Study the drawing (mm; zero at the part's minimum x, y, z) and answer. Round coordinates to 2 decimals unless told otherwise and drop trailing zeros. Write each loop counter-clockwise with the first axis right and the second up, starting at its lowest first coordinate (ties: lowest second). Pieces come first, ordered by that corner, then holes.
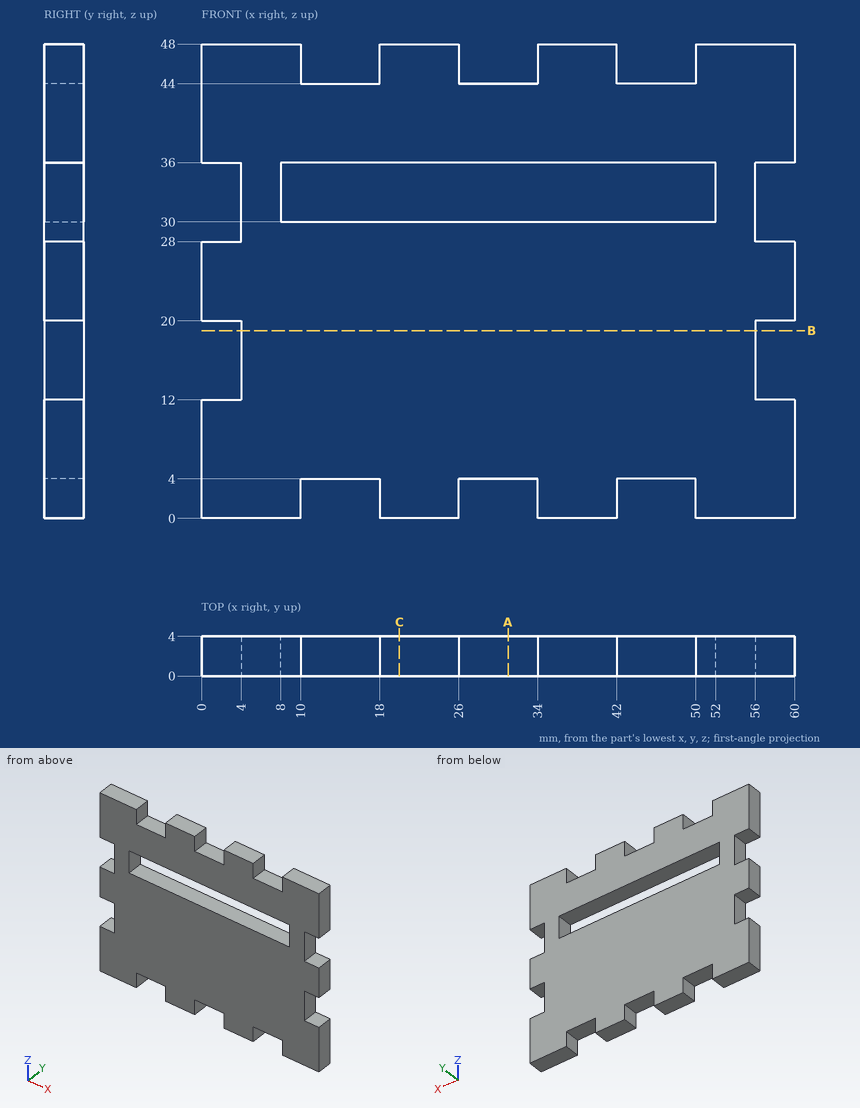
1. Section C-C on x = 20 is taken. Determine the outline of the cut face in (y, z).
Geometry says:
outline: (0, 0) - (4, 0) - (4, 30) - (0, 30) - close; (0, 36) - (4, 36) - (4, 48) - (0, 48) - close
2. Straight lines are drawn through the part: line 1 along X through (y, z) = (1, 46); line 2 along X through (y, z) = (1.3, 33); line 3 along Z through (x, y) = (48.5, 0.3). For each, find the intervals that lie inside material, in ascending order.
Geometry says:
line 1: x = 0 to 10, 18 to 26, 34 to 42, 50 to 60
line 2: x = 4 to 8, 52 to 56
line 3: z = 4 to 30, 36 to 44
3. Given pin 1 (1.5 mm diameter, centred on y = 3, z = 15.5, fed in from +X); pin 2 (1 mm diameter, centred on x = 45.5, y = 2, fed in from +Z); pin 3 (2 mm diameter, centred on y = 2, z = 16, fed in from -X), each flat-ended and moving along its own axis, determine where each tip first touches the part or whether it passes through.
Geometry says:
pin 1: stops at x = 56
pin 2: stops at z = 44
pin 3: stops at x = 4
4. Section A-A on x = 31 is taken. Determine the outline of the cut face in (y, z), plus the area to 3 significant figures.
Geometry says:
outline: (0, 4) - (4, 4) - (4, 30) - (0, 30) - close; (0, 36) - (4, 36) - (4, 44) - (0, 44) - close
area: 136 mm2
5. Section B-B on z = 19 is taken. Determine the outline of the cut face in (x, y), plus the area to 3 significant figures.
Geometry says:
outline: (4, 0) - (56, 0) - (56, 4) - (4, 4) - close
area: 208 mm2
